For this review, take the finished solid that the model builds, in its own axes (mm). A direction names the side the tool comes from. Give positions to 0.01 mm unless a question says otherwise; leave off trailing zeros. Write each loop counter-clockwise with the first axis right and the second up, starting at its lowest first coordinate (ties: lowest second). Pieces come first, ordered by that corner, then holes. Notation, with made-up numbers: (65.25, -11) -> (98.25, -11) arc R27 ccw to (98.25, 11) -> close; hole circle Ø8 at (44, 40). An arc over 180 degrees is marked (long way). Answer as CSV lines item,"result".
Autodesk Fusion 360 part; units mm, degrees
sketch "Sketch1" plane through (0, 0, 0) normal (0, 0, 1) x (1, 0, 0)
  line L0 (33, -21) -> (-33, -21)
  line L1 (-33, -21) -> (-33, 21)
  line L2 (-33, 21) -> (33, 21)
  line L3 (33, 21) -> (33, -21)
  line L4 (33, -21) -> (-33, 21) construction
  line L5 (-33, -21) -> (33, 21) construction
  dimension "d1" = 66
  dimension "d2" = 42
extrude "Extrude1" add sketch "Sketch1" along normal blind 12
chamfer "Chamfer1" distance 12 angle 45 2 edges at (33, -21, 6) (33, 21, 6)
sketch "Sketch2" plane through (0, 0, 12) normal (0, 0, 1) x (-1, 0, 0)
  line L0 (-33, -9) -> (-21, -21)
  line L1 (-21, -21) -> (33, -21)
  line L2 (33, -21) -> (33, 21)
  line L3 (33, 21) -> (-21, 21)
  line L4 (-21, 21) -> (-33, 9)
  line L5 (-33, 9) -> (-33, -9)
  line L6 (33, 21) -> (21, 21)
  line L7 (21, 21) -> (21, -21)
  line L8 (21, -21) -> (33, -21)
  line L9 (33, -21) -> (33, 21)
  dimension "d6" = 12
extrude "Extrude2" add sketch "Sketch2" along normal blind 48 contours L1 L2 L3 L6 L7 L8 L9
fillet "Fillet1" radius 21 2 edges at (-27, -21, 60) (-27, 21, 60)
sketch "Sketch6" plane through (0, 0, 0) normal (0, 1, 0) x (1, 0, 0)
  line L0 (-21, -49) -> (-21, -12)
  line L1 (-21, -12) -> (33, -12)
  line L2 (33, -12) -> (-21, -49)
  dimension "d11" = 37
extrude "Extrude3" add sketch "Sketch6" along normal mid plane 12
equation "d7 = 60 mm - 12 mm"
Q1. To check wall thickness, follow probe 1 along Z at (x, y) = (0.5, -10); probe 2 along Y at (x, z) = (16.5, 22.5); probe 3 along X at (y, z) = (-5.5, 57). State the ranges of each line that lie inside material, in increasing order. Write a range as [from, to].
Answer block:
probe 1,"z = [0, 12]"
probe 2,"y = [-6, 6]"
probe 3,"x = [-33, -21]"
Q2. Add section C-C (y = 15). Write out the cut boundary in (x, z).
Answer block:
outline,"(-33, 0) -> (27, 0) -> (27, 12) -> (-21, 12) -> (-21, 53.7) -> (-33, 53.7) -> close"
Q3. Add section A-A (z = 4.5). Write out the cut boundary in (x, y).
Answer block:
outline,"(-33, -21) -> (21, -21) -> (33, -9) -> (33, 9) -> (21, 21) -> (-33, 21) -> close"
Q4. For faces 1 (the flat face through (6.38, -0.08, 30.24)), 2 (the flat face through (-12, 21, 11)), 3 (the flat face through (-21, -10, 36)), 4 (the flat face through (0, 6, 26)), 5 (the flat face through (6, -13, 12)), list the 3-axis set-ups (+Z, -Z, +X, -X, +Y, -Y) from which the entire face can be reached by the end or side of a thin tool; tool diameter is ignored.
Answer block:
face 1,"+Z, +X, +Y, -Y"
face 2,"+Z, -Z, +X, -X, +Y"
face 3,"+Z, +X"
face 4,"+Z, +X, +Y"
face 5,"+Z, +X, -Y"
Q5. Clearance check with flat-ended pins moving along their axes: pin 1 (1 mm diameter, centred on x = -15.5, y = 9.5, fed in from +Z); pin 2 (6 mm diameter, centred on x = 15, y = -2.5, fed in from +Z); pin 3 (8 mm diameter, centred on x = 1.5, y = 7.5, fed in from +Z). State where each tip first meets the part, or that it passes through.
Answer block:
pin 1,"stops at z = 12"
pin 2,"stops at z = 26.39"
pin 3,"stops at z = 36.12"
Q6. Add section D-D (x = -20). Write out the cut boundary in (y, z), plus the area to 3 significant figures.
Answer block:
outline,"(-21, 0) -> (21, 0) -> (21, 12) -> (6, 12) -> (6, 48.31) -> (-6, 48.31) -> (-6, 12) -> (-21, 12) -> close"
area,"940 mm2"
Q7. Add section B-B (x = 6). Write out the cut boundary in (y, z).
Answer block:
outline,"(-21, 0) -> (21, 0) -> (21, 12) -> (6, 12) -> (6, 30.5) -> (-6, 30.5) -> (-6, 12) -> (-21, 12) -> close"
